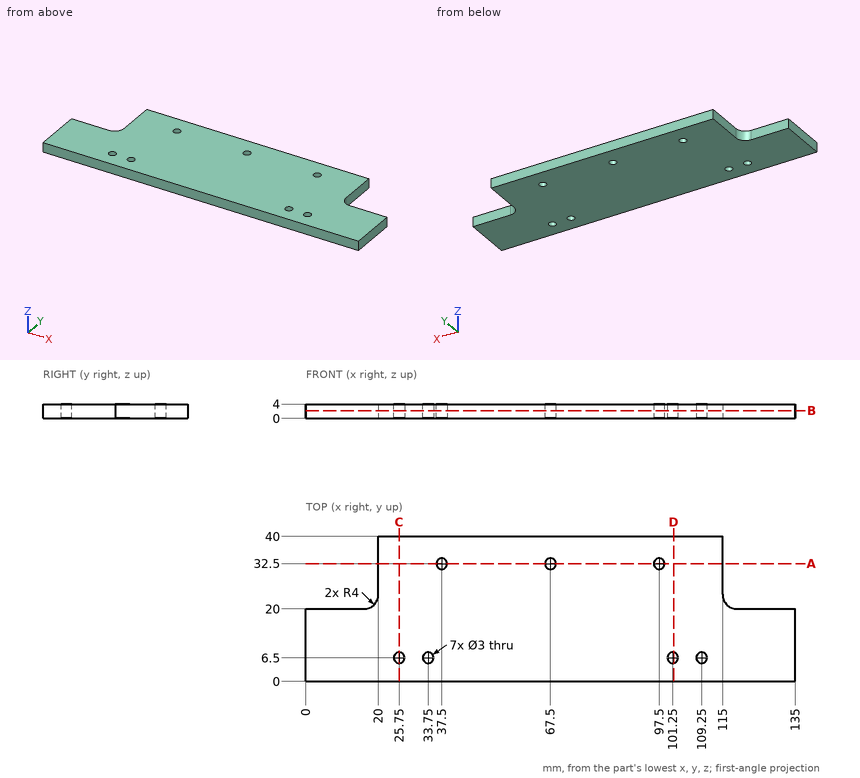
Answer from the drawing. Dimensions are ordinates in mm from the lowest x, y and z of the part. Coordinates: 2 decimals unless noted, no trailing zeros. Write each loop counter-clockwise with the first axis right and the second up, starting at its lowest first coordinate (ties: lowest second). Pieces come first, ordered by that corner, then holes. Notation, with made-up numbers: M 59,7 L 82,7 A16 ccw 82,28 Z; hole C 60.25,60.25 d2. An arc over 180 degrees is marked long. Write item = value, one per line.
1. The part is cut by section B-B (z = 2.2). Determine the outline of the cut face in (x, y).
Solution:
outline = M 0,0 L 135,0 L 135,20 L 119,20 A4 cw 115,24 L 115,40 L 20,40 L 20,24 A4 cw 16,20 L 0,20 Z; hole C 25.75,6.5 d3; hole C 33.75,6.5 d3; hole C 37.5,32.5 d3; hole C 67.5,32.5 d3; hole C 97.5,32.5 d3; hole C 101.25,6.5 d3; hole C 109.25,6.5 d3
2. The part is cut by section D-D (x = 101.5). Determine the outline of the cut face in (y, z), then the cut area to 3 significant figures.
Solution:
outline = M 0,0 L 5.02,0 L 5.02,4 L 0,4 Z; M 7.98,0 L 40,0 L 40,4 L 7.98,4 Z
area = 148 mm2
3. Straight lines are drawn through the part: line 1 (Y direction, x = 67.5, z = 1.65); line 2 (Y direction, x = 109.25, z = 1.95); line 3 (Y direction, x = 124, z = 3.45). For each, find the intervals that lie inside material, in ascending order. Write a range as from..to.
Solution:
line_1 = 0..31, 34..40
line_2 = 0..5, 8..40
line_3 = 0..20
4. The part is cut by section A-A (y = 32.5). Determine the outline of the cut face in (x, z), then the cut area to 3 significant figures.
Solution:
outline = M 20,0 L 36,0 L 36,4 L 20,4 Z; M 39,0 L 66,0 L 66,4 L 39,4 Z; M 69,0 L 96,0 L 96,4 L 69,4 Z; M 99,0 L 115,0 L 115,4 L 99,4 Z
area = 344 mm2
5. The part is cut by section C-C (x = 25.75). Determine the outline of the cut face in (y, z).
Solution:
outline = M 0,0 L 5,0 L 5,4 L 0,4 Z; M 8,0 L 40,0 L 40,4 L 8,4 Z
6. Flat-ended cylindrical pins translate along their axes: pin 1 (5 mm diameter, centred on x = 37.5, y = 32.5, fed in from -Z); pin 2 (1.8 mm diameter, centred on x = 67.5, y = 32.5, fed in from -Z); pin 3 (1.2 mm diameter, centred on y = 35.5, z = 1, fed in from -X); pin 4 (2 mm diameter, centred on y = 30, z = 1, fed in from +X). Find the tip coordinate at first contact, or state that the pin passes through.
Solution:
pin_1 = 0
pin_2 = through
pin_3 = 20
pin_4 = 115
